```python
from build123d import *

# Parameters (mm, degrees)
SKETCH3_OUTSIDE_W  = 40.796
SKETCH3_OUTSIDE_H  = 40.796
CUT_EXTRUDE5_DEPTH = 7.62


with BuildPart() as part:
    # Sketch1 → Revolve1 (revolve)
    with BuildSketch(Plane.XY):
        Polygon((0, 11.43), (-7.62, 11.43), (-7.62, 12.446), (-40.894, 12.446), (-40.894, 0), (19.05, 0), (19.05, 6.35), (0, 6.35), align=None)
    revolve(axis=Axis((-40.894, 0, 0), (1, 0, 0)))

    # Sketch3 outside → Cut-Extrude5 (cut)
    with BuildSketch(Plane(origin=(0, 0, 0), x_dir=(0, 0, -1), z_dir=(1, 0, 0))):
        Rectangle(SKETCH3_OUTSIDE_W, SKETCH3_OUTSIDE_H)
        Polygon((5.95753309, 10.31875), (-5.95753309, 10.31875), (-11.91506618, 0), (-5.95753309, -10.31875), (5.95753309, -10.31875), (11.91506618, 0), align=None, mode=Mode.SUBTRACT)
    extrude(amount=-CUT_EXTRUDE5_DEPTH, mode=Mode.SUBTRACT)


solid = part.part
```
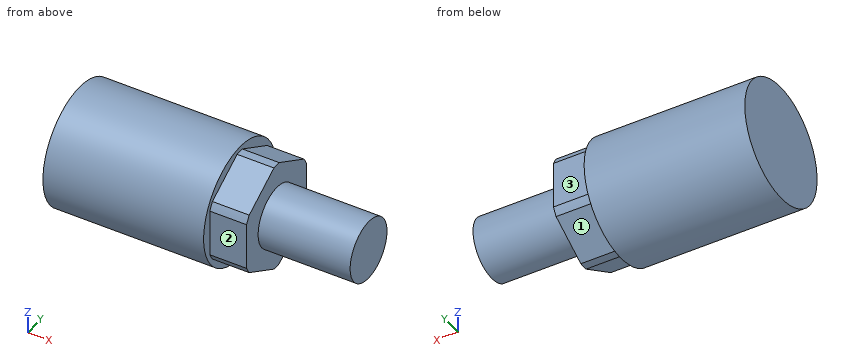
For this review, take the finished solid that the model builds, in its own axes (mm). Face numbers are marked on the shaded views. A direction names the side the tool comes from. Round coordinates to 2 decimals unless told otherwise and drop trailing zeros. Write each loop counter-clockwise with the first axis right and the second up, starting at its lowest first coordinate (ties: lowest second). Pieces come first, ordered by that corner, then holes. Notation, with made-up numbers: (42.5, -20.75) -> (60.5, -20.75) arc R26 cw to (60.5, 10.25) -> close; hole circle Ø7 at (29.25, 24). An arc over 180 degrees is marked (long way). Use one line per item in the form item = value.
1) To check wall thickness, follow L1, parallel to X at y = -8.5, z = -8.75; L2, parallel to X at y = 2.25, z = -9.5; L3, parallel to Y at x = 5, z = -0.25. State the ranges of each line that lie inside material, in increasing order. Write a range as from..to.
Found:
L1 = -40.89..-7.62
L2 = -40.89..0
L3 = -6.35..6.35
2) Take a section at C-C, the plane z = 7.25. Write out the cut boundary in (x, y), and give its area (3 significant figures).
Found:
outline = (-40.89, -10.12) -> (-7.62, -10.12) -> (-7.62, -8.08) -> (0, -8.08) -> (0, 8.08) -> (-7.62, 8.08) -> (-7.62, 10.12) -> (-40.89, 10.12) -> close
area = 796 mm2
3) Take a section at A-A, the plane y = 0. Write out the cut boundary in (x, z), and give its area (3 significant figures).
Found:
outline = (-40.89, -12.45) -> (-7.62, -12.45) -> (-7.62, -11.43) -> (0, -11.43) -> (0, -6.35) -> (19.05, -6.35) -> (19.05, 6.35) -> (0, 6.35) -> (0, 11.43) -> (-7.62, 11.43) -> (-7.62, 12.45) -> (-40.89, 12.45) -> close
area = 1,240 mm2
4) Take a section at B-B, the plane z = 0. Write out the cut boundary in (x, y), and give its area (3 significant figures).
Found:
outline = (-40.89, -12.45) -> (-7.62, -12.45) -> (-7.62, -10.32) -> (0, -10.32) -> (0, -6.35) -> (19.05, -6.35) -> (19.05, 6.35) -> (0, 6.35) -> (0, 10.32) -> (-7.62, 10.32) -> (-7.62, 12.45) -> (-40.89, 12.45) -> close
area = 1,230 mm2
5) Tool access review of the marked faces 1, 2 and 3: name each direction out of +Z, -Z, +X, -X, +Y, -Y from which nothing blocks a thin tool from reaching the whole face with its end or side.
Found:
face_1 = -Z, +X, +Y
face_2 = +Z, -Z, +X, -Y
face_3 = +Z, -Z, +X, +Y
6) Take a section at D-D, the plane y = 7.75. Write out the cut boundary in (x, z).
Found:
outline = (-40.89, -9.74) -> (-7.62, -9.74) -> (-7.62, -7.44) -> (0, -7.44) -> (0, 7.44) -> (-7.62, 7.44) -> (-7.62, 9.74) -> (-40.89, 9.74) -> close
7) Clearance check with flat-ended pins moving along their axes: pin 1 (4 mm diameter, centred on x = -4.5, z = -1.5, fed in from +Y); pin 2 (5 mm diameter, centred on x = -10.5, y = -4.5, fed in from +Z); pin 3 (2 mm diameter, centred on x = 11.5, y = -6.5, fed in from +Z); pin 4 (8.5 mm diameter, centred on x = -5, z = 1.5, fed in from -Y). State where each tip first meets the part, or that it passes through.
Found:
pin_1 = 10.32
pin_2 = 12.28
pin_3 = 3.17
pin_4 = -12.45
